For this review, use the dimensioned drawing (mm, ordinates from the lowest corner) and the shaded views. A direction names the side the tool comes from. Give positions to 0.01 mm unless a question says otherwise; leave off trailing zeros. Loops run counter-clockwise (first coordinate to the right, second up) from the corner with the lowest first, then second, coordinate; pieces in that order, holes last. Notation, with made-up numbers: (-29, 89.25) -> (-18, 89.25) arc R27 cw to (-18, 107.25) -> close; hole circle Ø10 at (-31.5, -15.75). An arc over 180 degrees is marked (long way). Use a Markdown table: item, result. Add a question column.
1. Draft analysis for pull direction Y (two halves, no side actions). For the marked faces 1, 2, 3 and 4, state which applies: pulls with the +Y half, pulls with the -Y half, needs draft (parallel to the pull), parting line crosses it, or undercut.
2. Add section A-A (x = 42). State the section outline as (y, z) points.
3. For the marked faces 5 and 6, list the 3-axis set-ups (+Z, -Z, +X, -X, +Y, -Y) from which the entire face can be reached by the end or side of a thin tool; tool diameter is ignored.
4. Add section C-C (z = 11.5). State the section outline as (x, y) points, and give its area (3 significant figures).
5. Add section D-D (z = 22). State the section outline as (x, y) points, and give its area (3 significant figures).
6. Add section B-B (y = 41). State the section outline as (x, z) points, and give its area (3 significant figures).
7. To check wall thickness, follow line 1 (Y direction, x = 49, z = 8.5); line 2 (Z direction, x = 59.5, y = 47.5); line 3 (X direction, y = 47, z = 28.5). State the ranges of each line that lie inside material, in increasing order.
8. For pin 1 Ø10 at (y, z) = (40.5, 21) entering from +X; pin 2 Ø1.5 at (x, y) = (54, 14.5) entering from +Z; pin 3 Ø6 at (y, z) = (45, 31.5) entering from -X, all flat-tipped, find the tip position at first contact; note any pin that passes through.
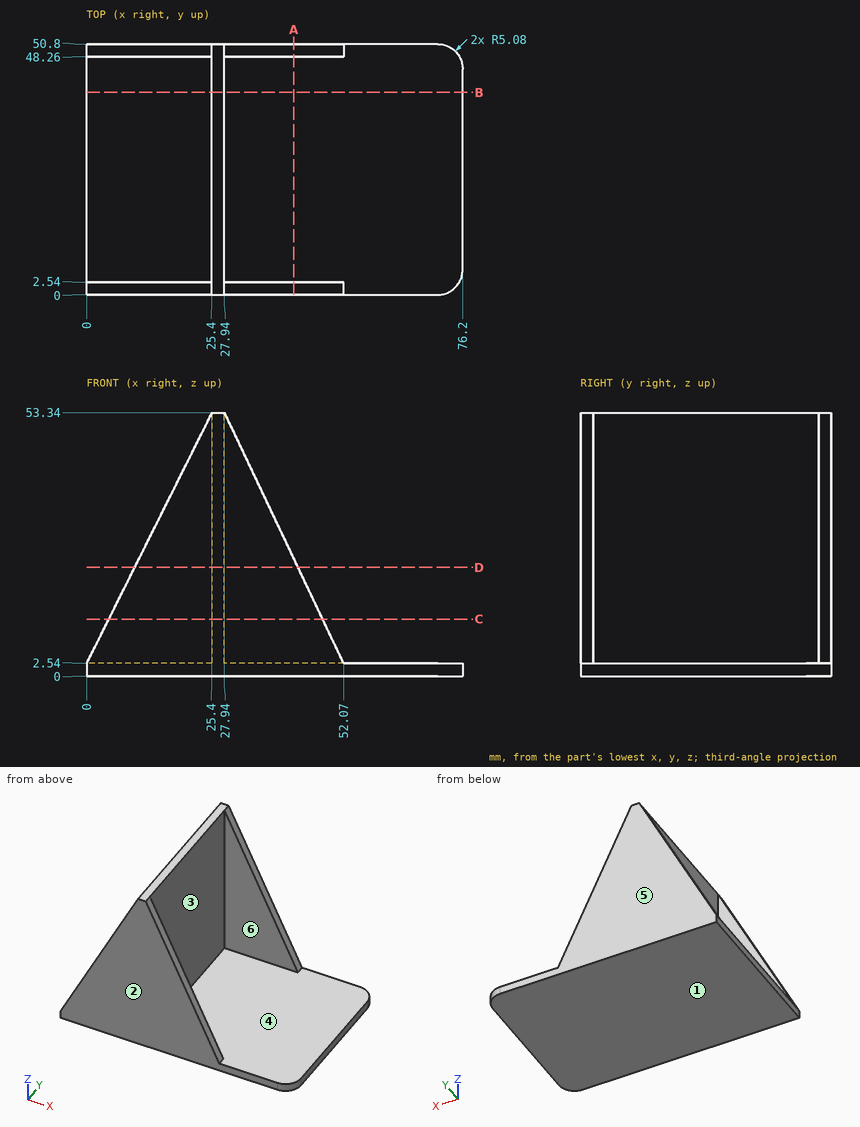
Taken from the geometry:
| question | item | result |
|---|---|---|
| 1 | face 1 | needs draft |
| 1 | face 2 | pulls with the -Y half |
| 1 | face 3 | undercut |
| 1 | face 4 | undercut |
| 2 | outline | (0, 0) -> (50.8, 0) -> (50.8, 23.74) -> (48.26, 23.74) -> (48.26, 2.54) -> (2.54, 2.54) -> (2.54, 23.74) -> (0, 23.74) -> close |
| 3 | face 5 | +Z, -Z, +X, -X, +Y |
| 3 | face 6 | +Z, +X |
| 4 | outline | (4.48, 0) -> (47.81, 0) -> (47.81, 2.54) -> (27.94, 2.54) -> (27.94, 48.26) -> (47.81, 48.26) -> (47.81, 50.8) -> (4.48, 50.8) -> (4.48, 48.26) -> (25.4, 48.26) -> (25.4, 2.54) -> (4.48, 2.54) -> close |
| 4 | area | 336 mm^2 |
| 5 | outline | (9.73, 0) -> (42.83, 0) -> (42.83, 2.54) -> (27.94, 2.54) -> (27.94, 48.26) -> (42.83, 48.26) -> (42.83, 50.8) -> (9.73, 50.8) -> (9.73, 48.26) -> (25.4, 48.26) -> (25.4, 2.54) -> (9.73, 2.54) -> close |
| 5 | area | 284 mm^2 |
| 6 | outline | (0, 0) -> (76.2, 0) -> (76.2, 2.54) -> (27.94, 2.54) -> (27.94, 53.34) -> (25.4, 53.34) -> (25.4, 2.54) -> (0, 2.54) -> close |
| 6 | area | 323 mm^2 |
| 7 | line 1 | y = 0 to 2.54, 48.26 to 50.8 |
| 7 | line 2 | z = 0 to 2.54 |
| 7 | line 3 | x = 25.4 to 27.94 |
| 8 | pin 1 | stops at x = 27.94 |
| 8 | pin 2 | stops at z = 2.54 |
| 8 | pin 3 | stops at x = 25.4 |
